Read the model definition and answer for the solid it produces. Units are mm, in the model's axes. Face numbers are marked on the shaded views. A direction names the side the tool comes from. Coordinates: 2 decimals unless noted, no trailing zeros. Write each loop counter-clockwise with the first axis right and the second up, starting at its lowest first coordinate (ties: lowest second). Pieces come first, ordered by that corner, then holes.
from build123d import *

# Parameters (mm, degrees)
SALIENTE_EXTRUIR1_DEPTH = 20
CORTAR_EXTRUIR1_START   = -10
CROQUIS2_R              = 4.7625
CORTAR_EXTRUIR1_DEPTH   = 10


with BuildPart() as part:
    # Croquis1 → Saliente-Extruir1 (new body)
    with BuildSketch(Plane.XY):
        Polygon((0, 0), (25, 0), (25, -2.5), (22.5, -2.5), (17.5, -10), (7.5, -10), (2.5, -2.5), (0, -2.5), align=None)
    extrude(amount=SALIENTE_EXTRUIR1_DEPTH)

    # Croquis2 → Cortar-Extruir1 (cut)
    with BuildSketch(Plane(origin=(0, 0, 0), x_dir=(1, 0, 0), z_dir=(0, 1, 0)).offset(CORTAR_EXTRUIR1_START)):
        with Locations(Location((12.5, -10, 0), (0, 0, 270))):
            Circle(CROQUIS2_R)
    extrude(amount=CORTAR_EXTRUIR1_DEPTH, mode=Mode.SUBTRACT)


solid = part.part
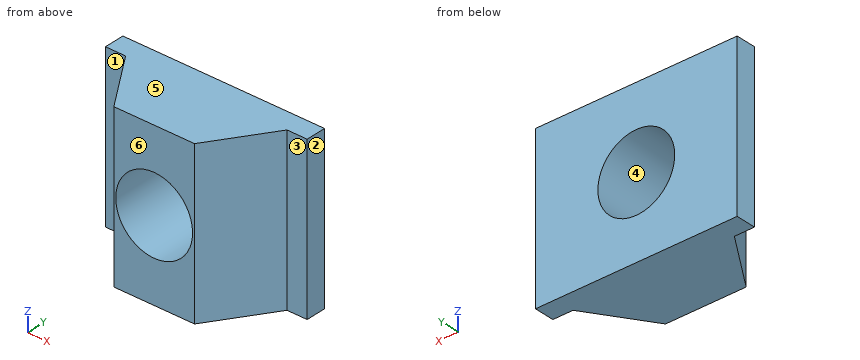
Item 1: Determine the mould class of the marked faces 4, 5 and 6 for opening direction Z: +Z half, -Z half, draft (parallel to the pull), parting line (faces both ways), or undercut.
Item 2: The part is cut by section D-D (z = 14.25). Give the vertices of the cut face in (x, y), and give its area (3 significant figures).
Item 3: Given pin 1 (5 mm diameter, centred on y = -8.5, z = 12, fed in from +X); pin 2 (1 mm diameter, centred on y = -4.5, z = 4, fed in from -X); pin 3 (2 mm diameter, centred on x = 1, z = 11.5, fed in from -Y), each flat-ended and moving along its own axis, determine where each tip first touches the part or whether it passes through.
Item 4: The part is cut by section C-C (y = -3.25). Give the vertices of the cut face in (x, z) (1 decimal).
Item 5: The part is cut by section A-A (x = 12.5). Give the vertices of the cut face in (y, z).
Item 6: Find the intervals of material crossed by probe 1 along X at (y, z) = (-2.25, 10); probe 2 along X at (y, z) = (-4.75, 10); probe 3 along Z at (x, y) = (11, -9), in increasing order.
Item 7: For the marked faces 1, 2 and 3, determine the directions among +Z, -Z, +X, -X, +Y, -Y from which every point of the face is accessible in a straight line to the end or side of a thin tool.
Item 8: The part is cut by section B-B (z = 10). Give the vertices of the cut face in (x, y).
Answer:
1. face 4: undercut
1. face 5: +Z half
1. face 6: draft
2. outline: (0, -2.5) - (2.5, -2.5) - (7.5, -10) - (10.35, -10) - (10.35, 0) - (0, 0) - close; (14.65, -10) - (17.5, -10) - (22.5, -2.5) - (25, -2.5) - (25, 0) - (14.65, 0) - close
2. area: 132 mm2
3. pin 1: stops at x = 20.17
3. pin 2: stops at x = 3.5
3. pin 3: stops at y = -2.5
4. outline: (3, 0) - (22, 0) - (22, 20) - (3, 20) - close; hole circle Ø9.5 at (12.5, 10)
5. outline: (-10, 0) - (0, 0) - (0, 5.24) - (-10, 5.24) - close; (-10, 14.76) - (0, 14.76) - (0, 20) - (-10, 20) - close
6. probe 1: x = 0 to 7.74, 17.26 to 25
6. probe 2: x = 4 to 7.74, 17.26 to 21
6. probe 3: z = 0 to 5.48, 14.52 to 20
7. face 1: +Z, -Z, -X, -Y
7. face 2: +Z, -Z, +X, +Y, -Y
7. face 3: +Z, -Z, +X, -Y
8. outline: (0, -2.5) - (2.5, -2.5) - (7.5, -10) - (7.74, -10) - (7.74, 0) - (0, 0) - close; (17.26, -10) - (17.5, -10) - (22.5, -2.5) - (25, -2.5) - (25, 0) - (17.26, 0) - close
